```python
from build123d import *

# Parameters (mm, degrees)
SKETCH1_W                = 13.2715
SKETCH1_H                = 80.00000002
SKETCH1_W_2              = 6.9215
SKETCH1_H_2              = 63.5
BOSS_EXTRUDE1_DEPTH      = 3.175
BOSS_EXTRUDE1_DEPTH_BACK = 6.35
SKETCH4_R                = 1.399999994
CUT_EXTRUDE1_DEPTH       = 81.00000002
CHAMFER1_SIZE            = 1.5875
CHAMFER1_SIZE2           = 0.916543552


with BuildPart() as part:
    # Sketch1 → Boss-Extrude1 (new body, two sides)
    with BuildSketch(Plane(origin=(0, 0, 0), x_dir=(1, 0, 0), z_dir=(0, 1, 0))) as boss_extrude1_sk:
        Rectangle(SKETCH1_W, SKETCH1_H)
        Rectangle(SKETCH1_W_2, SKETCH1_H_2, mode=Mode.SUBTRACT)
    extrude(amount=BOSS_EXTRUDE1_DEPTH)
    extrude(boss_extrude1_sk.sketch, amount=-BOSS_EXTRUDE1_DEPTH_BACK)

    # Sketch4 → Cut-Extrude1 (cut, through all)
    with BuildSketch(Plane.XY.offset(40.00000001)):
        Circle(SKETCH4_R)
    extrude(amount=-CUT_EXTRUDE1_DEPTH, mode=Mode.SUBTRACT)

    # Chamfer1
    chamfer1_edges = [part.edges().sort_by_distance(p)[0] for p in [
        (6.63575, -6.35, 0),
    ]]
    chamfer1_side = [part.faces().sort_by_distance(p)[0] for p in [
        (0, -6.35, 39.18906643),
    ]]
    chamfer(chamfer1_edges, length=CHAMFER1_SIZE, length2=CHAMFER1_SIZE2, reference=chamfer1_side[0])


solid = part.part
```
The listing builds one solid part. Answer for the finished solid, in the listing's coordinates (mm). A direction names the side the tool comes from. Coordinates: 2 decimals unless noted, no trailing zeros. Loops run counter-clockwise (first coordinate to the right, second up) from the corner with the lowest first, then second, coordinate; pieces in that order, holes last. Notation, with made-up numbers: (-4, -35) - (55, -35) arc R30 cw to (55, -11) - close; hole circle Ø9 at (40, -31.75). An arc over 180 degrees is marked (long way). Use a Markdown table: item, result. Add a question column.
1) For faces 4 (the cylindrical face through (-0.303, -1.367, -35.817)), 5 (the flat face through (3.461, -2, 0)), determine the directions among +Z, -Z, +X, -X, +Y, -Y from which every point of the face is accessible in a straight line to the end or side of a thin tool.
2) Find the intervals of material crossed by line 1 (Y direction, x = 0, z = 36.5) (3 decimals); line 2 (Z direction, x = 0.5, y = -2.25); line 3 (X direction, y = -3.5, z = -10), in increasing order.
3) The part is cut by section D-D, the plane z = 33. Give the vertices of the cut face in (x, y) (3 decimals), and give its area (3 significant figures).
4) The part is cut by section A-A, the plane z = -8.5. Give the vertices of the cut face in (x, y) (3 decimals), and give its area (3 significant figures).
5) The part is cut by section C-C, the plane y = -2.5. Give the vertices of the cut face in (x, z).
6) The part is cut by section B-B, the plane x = 0. Give the vertices of the cut face in (y, z) (3 decimals), and give its area (3 significant figures).
7) Given pin 1 (6 mm diameter, centred on x = -3, z = -6.5, fed in from +Y) (3 decimals); pin 2 (2.5 mm diameter, centred on x = 0, y = 0, fed in from +Z), each flat-ended and moving along its own axis, determine where each tip first touches the part or whether it passes through.
8) The mould has two halves that part along X. Classify faces 1 (the flat face through (6.636, -1, 1)), 2 (the flat face through (0, -2, -31.75)), 3 (the flat face through (0, -2, 40)): released by +X, released by -X, zero draft, split by the parting line, or undercut.
Here are the results:
| question | item | result |
|---|---|---|
| 1 | face 4 | +Z, -Z |
| 1 | face 5 | +Y, -Y |
| 2 | line 1 | y = -6.35 to -1.4, 1.4 to 3.175 |
| 2 | line 2 | z = -40 to -31.75, 31.75 to 40 |
| 2 | line 3 | x = -6.64 to -3.46, 3.46 to 6.64 |
| 3 | outline | (-6.636, -6.35) - (5.048, -6.35) - (6.636, -5.433) - (6.636, 3.175) - (-6.636, 3.175) - close; hole circle Ø2.8 at (0, 0) |
| 3 | area | 120 mm^2 |
| 4 | outline | (-6.636, -6.35) - (-3.461, -6.35) - (-3.461, 3.175) - (-6.636, 3.175) - close; (3.461, -6.35) - (5.048, -6.35) - (6.636, -5.433) - (6.636, 3.175) - (3.461, 3.175) - close |
| 4 | area | 59.8 mm^2 |
| 5 | outline | (-6.64, -40) - (6.64, -40) - (6.64, 40) - (-6.64, 40) - close; hole (-3.46, -31.75) - (3.46, -31.75) - (3.46, 31.75) - (-3.46, 31.75) - close |
| 6 | outline | (-6.35, -40) - (-1.4, -40) - (-1.4, -31.75) - (-6.35, -31.75) - close; (-6.35, 31.75) - (-1.4, 31.75) - (-1.4, 40) - (-6.35, 40) - close; (1.4, -40) - (3.175, -40) - (3.175, -31.75) - (1.4, -31.75) - close; (1.4, 31.75) - (3.175, 31.75) - (3.175, 40) - (1.4, 40) - close |
| 6 | area | 111 mm^2 |
| 7 | pin 1 | stops at y = 3.175 |
| 7 | pin 2 | passes through |
| 8 | face 1 | released by +X |
| 8 | face 2 | undercut |
| 8 | face 3 | zero draft |
